```python
from build123d import *

# Parameters (mm, degrees)
F0_R   = 53
F0_R_2 = 51.5


with BuildPart() as f2:
    # F2: sweep along a path in F1
    with BuildLine(Plane.YZ) as f2_path:
        Line((0, 0), (-44, 0))
        ThreePointArc((-44, 0), (-118.953319, -31.046681), (-150, -106))
        Line((-150, -106), (-150, -394))
        ThreePointArc((-150, -394), (-181.046681, -468.953319), (-256, -500))
        Line((-256, -500), (-650, -500))
    # F0 (on Front) → F2 (sweep)
    with BuildSketch(Plane.XZ):
        Circle(F0_R)
        Circle(F0_R_2, mode=Mode.SUBTRACT)
    sweep(path=f2_path.line)


solid = f2.part
```
The listing builds one solid part. Answer for the finished solid, in the listing's coordinates (mm). A direction names the side the tool comes from. Coordinates: 2 decimals unless noted, no trailing zeros. Write each loop counter-clockwise with the first axis right and the second up, starting at its lowest first coordinate (ties: lowest second). Pieces come first, ordered by that corner, then holes. Notation, with made-up numbers: M 42,33.25 L 46,33.25 A5 ccw 46,38.25 Z; hole C -2,-2 d3. An arc over 180 degrees is marked long. Use a Markdown table: item, result. Add a question column.
1. Straight lines are drawn through the part: line 1 along Y through (x, z) = (-0.5, -194); line 2 along Z through (x, y) = (0, -546); line 3 along Z through (x, y) = (0, -20.5). For each, find the intervals that lie inside material, in ascending order. Write a range as [from, to].
2. For a pull along Z with two mould halves and no side action, classify faces 4 (the flat face through (51.3, -650, -491.9)), 5 (the cylindrical face through (24.46, -455.76, -547.02)), 6 (the cylindrical face through (-11.164, -22.308, -50.275)) as +Z half, -Z half, draft (parallel to the pull), parting line (faces both ways), or undercut.
3. Which of the six approach directions +Z, -Z, +X, -X, +Y, -Y give full straight-line access (tool end or side, diameter ignored) to faces 1 (the flat face through (51.3, 0, 8.1)), 2 (the cylindrical face through (28, -22, 45)), 3 (the cylindrical face through (-6.704, -455.758, -448.938))?
4. Given P1, Ø10, axis at x = 26.5, y = -196, coming from the -Z side; P2, Ø6, axis at x = 35.5, z = -55, coming from the +Y side; P3, Ø1.5, axis at x = -10.5, y = -575.5, coming from the -Z side, each flat-ended and moving along its own axis, determine where each tip first touches the part or whether it passes through.
5. Section A-A (y = -514.5) is taken. Give the vertices of the cut face in (x, z).
Data:
| question | item | result |
|---|---|---|
| 1 | line 1 | y = [-203, -201.5], [-98.5, -97] |
| 1 | line 2 | z = [-553, -551.5], [-448.5, -447] |
| 1 | line 3 | z = [-53, -51.5], [51.5, 53] |
| 2 | face 4 | draft |
| 2 | face 5 | parting line |
| 2 | face 6 | undercut |
| 3 | face 1 | +Z, -Z, +X, -X, +Y |
| 3 | face 2 | +Y |
| 3 | face 3 | -Y |
| 4 | P1 | stops at z = -537.05 |
| 4 | P2 | stops at y = -81.16 |
| 4 | P3 | stops at z = -552.1 |
| 5 | outline | C 0,-500 d106; hole C 0,-500 d103 |
